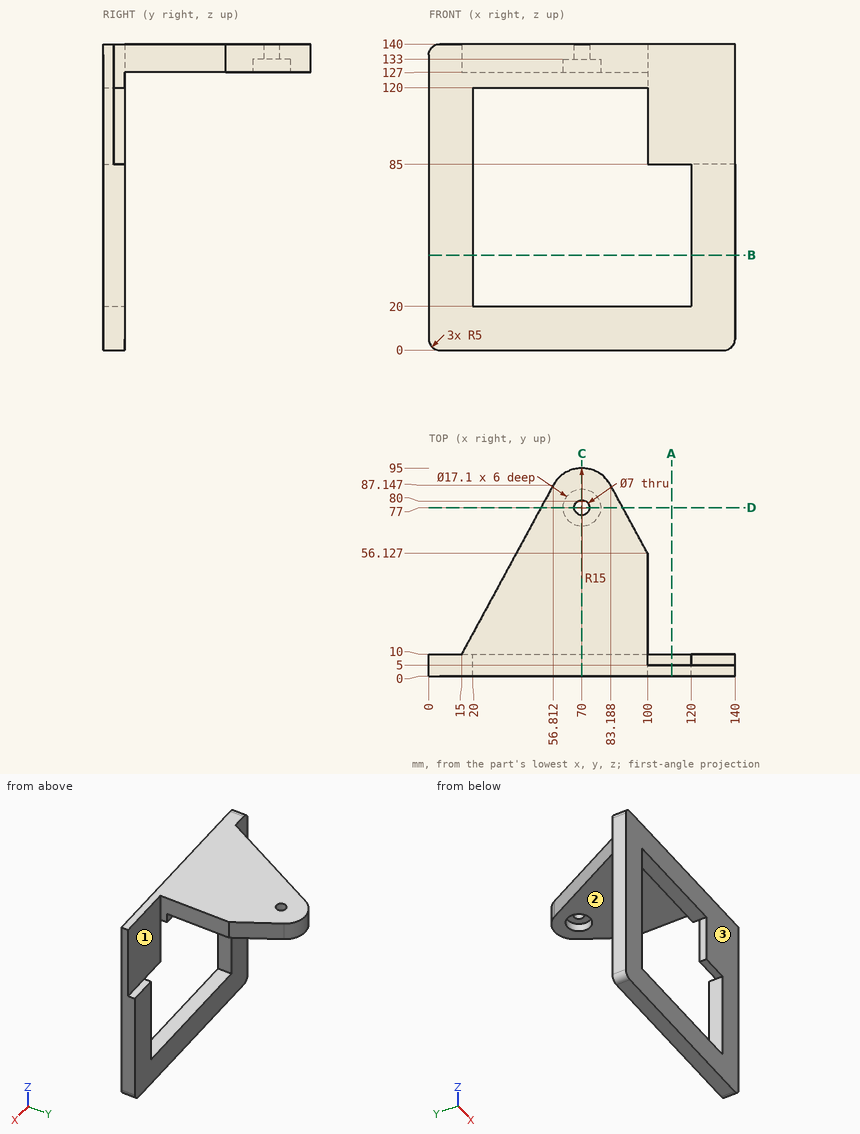
Geometry check sheet. Reference: drawing and pictorial views, mm from the part's lowest x, y, z. Coordinates: 2 decimals unless noted, no trailing zeros. Write each loop counter-clockwise with the first axis right and the second up, starting at its lowest first coordinate (ties: lowest second). Pieces come first, ordered by that corner, then holes. Notation, with made-up numbers: M -25,27 L 2,27 A36 cw 2,64 Z; hole C 88.5,-25.75 d4. An arc over 180 degrees is marked long. One line per question, with ' | ' between items.
1) Sectioned sample at C-C on x = 70. Record the cut outline in (y, z), then the cut area to 3 significant figures.
Solutions:
outline: M 0,0 L 10,0 L 10,20 L 0,20 Z; M 0,120 L 10,120 L 10,127 L 68.45,127 L 68.45,133 L 73.5,133 L 73.5,140 L 0,140 Z; M 80.5,133 L 85.55,133 L 85.55,127 L 95,127 L 95,140 L 80.5,140 Z | area: 1,350 mm^2
2) Sectioned sample at D-D on y = 77. Record the cut outline in (x, z).
Solutions:
outline: M 51.31,127 L 61.45,127 L 61.45,133 L 66.5,133 L 66.5,140 L 51.31,140 Z; M 73.5,133 L 78.55,133 L 78.55,127 L 88.69,127 L 88.69,140 L 73.5,140 Z
3) Depth check by flat-ended pin: pin 1 Ø8 at (x, y) = (70, 77) entering from +Z; pin 2 Ø5 at (x, z) = (44.5, 15.5) entering from +Y; pin 3 Ø10 at (y, z) = (19.5, 133) entering from +X; pin 4 Ø1.5 at (x, y) = (129, 6.5) entering from +Z. Enter the tip coordinate at first touch or a pass-through.
Solutions:
pin 1: z = 140 | pin 2: y = 10 | pin 3: x = 100 | pin 4: z = 85
4) Sectioned sample at A-A on x = 111. Record the cut outline in (y, z), then the cut area to 3 significant figures.
Solutions:
outline: M 0,0 L 10,0 L 10,20 L 0,20 Z; M 0,85 L 5,85 L 5,140 L 0,140 Z | area: 475 mm^2
5) Sectioned sample at B-B on z = 43.5. Record the cut outline in (x, y), then the cut area to 3 significant figures.
Solutions:
outline: M 0,0 L 20,0 L 20,10 L 0,10 Z; M 120,0 L 140,0 L 140,10 L 120,10 Z | area: 400 mm^2
6) Release check for a two-part mould opening along Y. For the marked faces 1, 2 and 3 record: +Y half, -Y half, draft (parallel to the pull), parting line (faces both ways), or undercut.
Solutions:
face 1: +Y half | face 2: draft | face 3: -Y half
7) Material ranges on L1, parallel to Y at x = 70, z = 136; L2, parallel to Y at x = 70, z = 131.05; L3, parallel to Y at x = 119.5, z = 15, recorded low to high.
Solutions:
L1: 0 to 73.5, 80.5 to 95 | L2: 0 to 68.45, 85.55 to 95 | L3: 0 to 10
